```python
from build123d import *

# Parameters (mm, degrees)
SKETCH2_W             = 219
SKETCH2_H             = 105
BOSS_EXTRUDE1_DEPTH   = 2.5
SKETCH3_W             = 219
SKETCH3_H             = 105
SKETCH3_W_2           = 214
SKETCH3_H_2           = 100
BOSS_EXTRUDE2_DEPTH   = 10
SKETCH5_R             = 3
BOSS_EXTRUDE3_DEPTH   = 23
M3_TAPPED_HOLE1_D     = 2.5
M3_TAPPED_HOLE1_DEPTH = 10.1
M3_TAPPED_HOLE1_TIP   = 0.751075774
SKETCH8_R             = 2
CUT_EXTRUDE1_DEPTH    = 10
VENT1_START           = -34.039390763
VENT1_OUTLINE_W       = 1.5
VENT1_OUTLINE_H       = 26
VENT1_DEPTH           = 26
VENT1_2_OUTLINE_W     = 1
VENT1_2_OUTLINE_H     = 4.25
VENT1_2_OUTLINE_H_2   = 5.25
VENT1_2_OUTLINE_H_3   = 3.5
VENT1_2_DEPTH         = 5.25
VENT1_START_2         = -12.289390763
VENT1_3_OUTLINE_W     = 1
VENT1_3_OUTLINE_H     = 4.25
VENT1_3_OUTLINE_H_2   = 5.25
VENT1_3_OUTLINE_H_3   = 3.5
VENT1_3_DEPTH         = 4.25
VENT1_START_3         = -27.289390763
VENT1_4_OUTLINE_W     = 1
VENT1_4_OUTLINE_H     = 4.25
VENT1_4_OUTLINE_H_2   = 5.25
VENT1_4_OUTLINE_H_3   = 3.5
VENT1_4_DEPTH         = 3.5
VENT1_START_4         = -22.289390763
VENT1_5_OUTLINE_W     = 1
VENT1_5_OUTLINE_H     = 4.25
VENT1_5_OUTLINE_H_2   = 5.25
VENT1_5_OUTLINE_H_3   = 3.5
VENT1_5_DEPTH         = 3.5
VENT1_START_5         = -17.289390763
VENT1_6_OUTLINE_W     = 1
VENT1_6_OUTLINE_H     = 4.25
VENT1_6_OUTLINE_H_2   = 5.25
VENT1_6_OUTLINE_H_3   = 3.5
VENT1_6_DEPTH         = 3.5
BOSS_EXTRUDE4_DEPTH   = 2.5
BOSS_EXTRUDE5_DEPTH   = 2.5
SKETCH13_W            = 121.7
SKETCH13_H            = 3
CUT_EXTRUDE2_DEPTH    = 10
SKETCH14_W            = 125.7
SKETCH14_H            = 1.05
CUT_EXTRUDE3_DEPTH    = 5


# Read off the part's stored shape, not the designer's step: Vent1
with BuildPart() as part:
    # Sketch2 → Boss-Extrude1 (new body)
    with BuildSketch(Plane(origin=(0, 0, 0), x_dir=(1, 0, 0), z_dir=(0, 1, 0))):
        Rectangle(SKETCH2_W, SKETCH2_H)
    extrude(amount=BOSS_EXTRUDE1_DEPTH)

    # Sketch3 → Boss-Extrude2 (add)
    with BuildSketch(Plane.XZ):
        Rectangle(SKETCH3_W, SKETCH3_H)
        Rectangle(SKETCH3_W_2, SKETCH3_H_2, mode=Mode.SUBTRACT)
    extrude(amount=BOSS_EXTRUDE2_DEPTH)

    # Sketch5 → Boss-Extrude3 (add)
    with BuildSketch(Plane.XZ):
        with Locations(Location((103, -46.5, 0), (0, 0, 90))):
            Circle(SKETCH5_R)
        with Locations(Location((-103, -46.5, 0), (0, 0, 90))):
            Circle(SKETCH5_R)
        with Locations(Location((-103, 46.5, 0), (0, 0, 90))):
            Circle(SKETCH5_R)
        with Locations(Location((103, 46.5, 0), (0, 0, 90))):
            Circle(SKETCH5_R)
    extrude(amount=BOSS_EXTRUDE3_DEPTH)

    # M3 Tapped Hole1
    with Locations(Plane(origin=(0, -23, 0), x_dir=(-1, 0, 0), z_dir=(0, -1, 0))):
        with Locations((-103, 46.5), (103, 46.5), (103, -46.5), (-103, -46.5)):
            Hole(M3_TAPPED_HOLE1_D / 2, depth=M3_TAPPED_HOLE1_DEPTH)
            with Locations((0, 0, -(M3_TAPPED_HOLE1_DEPTH + M3_TAPPED_HOLE1_TIP / 2))):  # 118° drill point
                Cone(0, M3_TAPPED_HOLE1_D / 2, M3_TAPPED_HOLE1_TIP, mode=Mode.SUBTRACT)

    # Sketch8 → Cut-Extrude1 (cut)
    with BuildSketch(Plane(origin=(0, 2.5, 0), x_dir=(1, 0, 0), z_dir=(0, 1, 0))):
        with Locations(Location((-5.039390763, -16, 0), (0, 0, 270))):
            Circle(SKETCH8_R)
        with Locations(Location((-37.039390763, -16, 0), (0, 0, 270))):
            Circle(SKETCH8_R)
        with Locations(Location((-37.039390763, 16, 0), (0, 0, 270))):
            Circle(SKETCH8_R)
        with Locations(Location((-5.039390763, 16, 0), (0, 0, 270))):
            Circle(SKETCH8_R)
    extrude(amount=-CUT_EXTRUDE1_DEPTH, mode=Mode.SUBTRACT)

    # Vent1 outline → Vent1 (cut)
    with BuildSketch(Plane.YZ.offset(VENT1_START)):
        with Locations((0.75, 0)):
            Rectangle(VENT1_OUTLINE_W, VENT1_OUTLINE_H)
    extrude(amount=VENT1_DEPTH, mode=Mode.SUBTRACT)

    # Vent1 2 outline → Vent1 2 (cut)
    with BuildSketch(Plane.YZ.offset(VENT1_START)):
        with Locations((2, 10.875)):
            Rectangle(VENT1_2_OUTLINE_W, VENT1_2_OUTLINE_H)
        with Locations((2, -10.375)):
            Rectangle(VENT1_2_OUTLINE_W, VENT1_2_OUTLINE_H_2)
        with Locations((2, 5.5)):
            Rectangle(VENT1_2_OUTLINE_W, VENT1_2_OUTLINE_H_3)
        with Locations((2, -4.5)):
            Rectangle(VENT1_2_OUTLINE_W, VENT1_2_OUTLINE_H_3)
        with Locations((2, 0.5)):
            Rectangle(VENT1_2_OUTLINE_W, VENT1_2_OUTLINE_H_3)
    extrude(amount=VENT1_2_DEPTH, mode=Mode.SUBTRACT)

    # Vent1 3 outline → Vent1 3 (cut)
    with BuildSketch(Plane.YZ.offset(VENT1_START_2)):
        with Locations((2, 10.875)):
            Rectangle(VENT1_3_OUTLINE_W, VENT1_3_OUTLINE_H)
        with Locations((2, -10.375)):
            Rectangle(VENT1_3_OUTLINE_W, VENT1_3_OUTLINE_H_2)
        with Locations((2, 5.5)):
            Rectangle(VENT1_3_OUTLINE_W, VENT1_3_OUTLINE_H_3)
        with Locations((2, -4.5)):
            Rectangle(VENT1_3_OUTLINE_W, VENT1_3_OUTLINE_H_3)
        with Locations((2, 0.5)):
            Rectangle(VENT1_3_OUTLINE_W, VENT1_3_OUTLINE_H_3)
    extrude(amount=VENT1_3_DEPTH, mode=Mode.SUBTRACT)

    # Vent1 4 outline → Vent1 4 (cut)
    with BuildSketch(Plane.YZ.offset(VENT1_START_3)):
        with Locations((2, 10.875)):
            Rectangle(VENT1_4_OUTLINE_W, VENT1_4_OUTLINE_H)
        with Locations((2, -10.375)):
            Rectangle(VENT1_4_OUTLINE_W, VENT1_4_OUTLINE_H_2)
        with Locations((2, 5.5)):
            Rectangle(VENT1_4_OUTLINE_W, VENT1_4_OUTLINE_H_3)
        with Locations((2, -4.5)):
            Rectangle(VENT1_4_OUTLINE_W, VENT1_4_OUTLINE_H_3)
        with Locations((2, 0.5)):
            Rectangle(VENT1_4_OUTLINE_W, VENT1_4_OUTLINE_H_3)
    extrude(amount=VENT1_4_DEPTH, mode=Mode.SUBTRACT)

    # Vent1 5 outline → Vent1 5 (cut)
    with BuildSketch(Plane.YZ.offset(VENT1_START_4)):
        with Locations((2, 10.875)):
            Rectangle(VENT1_5_OUTLINE_W, VENT1_5_OUTLINE_H)
        with Locations((2, -10.375)):
            Rectangle(VENT1_5_OUTLINE_W, VENT1_5_OUTLINE_H_2)
        with Locations((2, 5.5)):
            Rectangle(VENT1_5_OUTLINE_W, VENT1_5_OUTLINE_H_3)
        with Locations((2, -4.5)):
            Rectangle(VENT1_5_OUTLINE_W, VENT1_5_OUTLINE_H_3)
        with Locations((2, 0.5)):
            Rectangle(VENT1_5_OUTLINE_W, VENT1_5_OUTLINE_H_3)
    extrude(amount=VENT1_5_DEPTH, mode=Mode.SUBTRACT)

    # Vent1 6 outline → Vent1 6 (cut)
    with BuildSketch(Plane.YZ.offset(VENT1_START_5)):
        with Locations((2, 10.875)):
            Rectangle(VENT1_6_OUTLINE_W, VENT1_6_OUTLINE_H)
        with Locations((2, -10.375)):
            Rectangle(VENT1_6_OUTLINE_W, VENT1_6_OUTLINE_H_2)
        with Locations((2, 5.5)):
            Rectangle(VENT1_6_OUTLINE_W, VENT1_6_OUTLINE_H_3)
        with Locations((2, -4.5)):
            Rectangle(VENT1_6_OUTLINE_W, VENT1_6_OUTLINE_H_3)
        with Locations((2, 0.5)):
            Rectangle(VENT1_6_OUTLINE_W, VENT1_6_OUTLINE_H_3)
    extrude(amount=VENT1_6_DEPTH, mode=Mode.SUBTRACT)

    # Sketch10 → Boss-Extrude4 (add)
    with BuildSketch(Plane.XY.offset(52.5)):
        with BuildLine():
            Line((18.22, -16.75), (22.72, -16.75))
            Line((22.72, -16.75), (22.72, -9.51))
            Line((22.72, -9.51), (-56.08, -9.51))
            Line((-56.08, -9.51), (-56.08, -16.75))
            Line((-56.08, -16.75), (-51.08, -16.75))
            ThreePointArc((-51.08, -16.75), (-46.43, -12.1), (-41.78, -16.75))
            Line((-41.78, -16.75), (-36.08, -16.75))
            ThreePointArc((-36.08, -16.75), (-31.43, -12.1), (-26.78, -16.75))
            Line((-26.78, -16.75), (-21.08, -16.75))
            ThreePointArc((-21.08, -16.75), (-16.43, -12.1), (-11.78, -16.75))
            Line((-11.78, -16.75), (-6.08, -16.75))
            ThreePointArc((-6.08, -16.75), (-1.43, -12.1), (3.22, -16.75))
            Line((3.22, -16.75), (8.92, -16.75))
            ThreePointArc((8.92, -16.75), (13.57, -12.1), (18.22, -16.75))
        make_face()
    extrude(amount=-BOSS_EXTRUDE4_DEPTH)

    # Sketch12 → Boss-Extrude5 (add)
    with BuildSketch(Plane.XY.offset(52.5)):
        Polygon((99, -10), (99, -12.35), (89.6, -12.35), (89.6, -16.75), (34.8, -16.75), (34.8, -12.65), (24.85, -12.65), (24.85, -16.75), (22.72, -16.75), (22.72, -10), align=None)
    extrude(amount=-BOSS_EXTRUDE5_DEPTH)

    # Sketch13 → Cut-Extrude2 (cut)
    with BuildSketch(Plane(origin=(0, 0, -52.5), x_dir=(-1, 0, 0), z_dir=(0, 0, -1))):
        with Locations((-5.19, -8.5)):
            Rectangle(SKETCH13_W, SKETCH13_H)
    extrude(amount=-CUT_EXTRUDE2_DEPTH, mode=Mode.SUBTRACT)

    # Sketch14 → Cut-Extrude3 (cut)
    with BuildSketch(Plane.XZ.offset(10)):
        with Locations((5.19, -51.25)):
            Rectangle(SKETCH14_W, SKETCH14_H)
    extrude(amount=-CUT_EXTRUDE3_DEPTH, mode=Mode.SUBTRACT)


solid = part.part
```
The listing builds one solid part. Answer for the finished solid, in the listing's coordinates (mm). A direction names the side the tool comes from. Round coordinates to 2 decimals unless told otherwise and drop trailing zeros. Loops run counter-clockwise (first coordinate to the right, second up) from the corner with the lowest first, then second, coordinate; pieces in that order, holes last.
Q1. Which of the six approach directions +Z, -Z, +X, -X, +Y, -Y give full straight-line access (tool end or side, diameter ignored) to faces 4 (the face through (-100.07, -11.34, -47.15)), 5 (the face through (-103, -23, -45))?
Q2. Section A-A, the plane y = -2.5 is taken. Determine the outline of the cut face in (x, z).
Q3. Section D-D, the plane z = -16 is taken. Determine the outline of the cut face in (x, y).
Q4. Section B-B, the plane x = -31.43 is taken. Count the separate pieces of the cut face and the enclosed holes in it, then the cut area to 3 significant figures.
Q5. Find the intervals of material crossed by line 1 (X direction, y = -18, z = -46.5); line 2 (X direction, y = 1.45, z = 16); line 3 (X direction, y = -1.5, z = -47), in increasing order.
Q6. For a pull along Z with two mould halves and no side action, classify faces 1 (the face through (-100.07, -11.34, 45.85)), 2 (the face through (103, -23, -45)), 3 (the face through (2, -5, 52.5)) as released by +Z, released by -Z, zero draft, split by the parting line, or undercut.
Q7. Section C-C, the plane y = -20.75 is taken. Determine the outline of the cut face in (x, z), then the cut area to 3 significant figures.
Q8. Given pin 1 Ø5 at (x, z) = (-28.5, -38.5) entering from -Y; pin 2 Ø0.8 at (x, z) = (-23, 50.5) entering from -Y, each flat-ended and moving along its own axis, determine where each tip first touches the part or whether it passes through.
Completed:
1. face 4: -Y
1. face 5: +Z, -Z, +X, -X, -Y
2. outline: (-109.5, -52.5) - (109.5, -52.5) - (109.5, 52.5) - (-109.5, 52.5) - close; circle Ø6 at (-103, -46.5); circle Ø6 at (-103, 46.5); circle Ø6 at (103, -46.5); circle Ø6 at (103, 46.5); hole (-107, -50) - (107, -50) - (107, 50) - (-107, 50) - close
3. outline: (-109.5, -10) - (-107, -10) - (-107, 0) - (-39.04, 0) - (-39.04, 2.5) - (-109.5, 2.5) - close; (-35.04, 0) - (-7.04, 0) - (-7.04, 2.5) - (-35.04, 2.5) - close; (-3.04, 0) - (107, 0) - (107, -10) - (109.5, -10) - (109.5, 2.5) - (-3.04, 2.5) - close
4. separate pieces: 6
4. enclosed holes: 0
4. area: 249 mm2
5. line 1: x = -106 to -104.25, -101.75 to -100, 100 to 101.75, 104.25 to 106
5. line 2: x = -109.5 to -39.04, -35.04 to -7.04, -3.04 to 109.5
5. line 3: x = -109.5 to -107, -105.96 to -100.04, 100.04 to 105.96, 107 to 109.5
6. face 1: undercut
6. face 2: zero draft
6. face 3: released by +Z
7. outline: circle Ø6 at (-103, -46.5); circle Ø6 at (-103, 46.5); circle Ø6 at (103, -46.5); circle Ø6 at (103, 46.5); hole circle Ø2.5 at (-103, -46.5); hole circle Ø2.5 at (-103, 46.5); hole circle Ø2.5 at (103, -46.5); hole circle Ø2.5 at (103, 46.5)
7. area: 93.5 mm2
8. pin 1: stops at y = 0
8. pin 2: stops at y = -16.75
